Work out the finished part from the listing and answer in its coordinate system (mm). A direction names the side the tool comes from. Give positions to 0.01 mm unless a question says otherwise; leave off trailing zeros. Loops run counter-clockwise (first coordinate to the right, second up) from the corner with the lowest first, then second, coordinate; pieces in that order, holes last. Notation, with made-up numbers: M 58,13.25 L 87,13.25 A26 ccw 87,28.25 Z; hole C 58,12 d5. An arc over 180 degrees is marked long. Answer in a Markdown table with one row per item. Add a question column.
from build123d import *

# Parameters (mm, degrees)
F0_W      = 131
F0_H      = 59
F0_W_2    = 85
F0_H_2    = 55
F0_W_3    = 40
F1_DEPTH  = 22
F2_W      = 40
F2_H      = 2
F3_DEPTH  = 55
F4_W      = 85
F4_H      = 3.4782900475
F5_DEPTH  = 55
F7_DEPTH  = 2
F8_R      = 2
F9_DEPTH  = 2
F10_R     = 4
F11_DEPTH = 20
F12_DEPTH = 20
F13_R     = 4
F14_R     = 6.25
F15_DEPTH = 25


with BuildPart() as f1:
    # F0 (on Top) → F1 (new body)
    with BuildSketch(Plane.XY):
        Rectangle(F0_W, F0_H)
        with Locations((-21, 0)):
            Rectangle(F0_W_2, F0_H_2, mode=Mode.SUBTRACT)
        with Locations((43.5, 0)):
            Rectangle(F0_W_3, F0_H_2, mode=Mode.SUBTRACT)
    extrude(amount=F1_DEPTH)

    # F2 (on face) → F3 (join)
    with BuildSketch(Plane.XZ.offset(-27.5)):
        with Locations((43.5, 21)):
            Rectangle(F2_W, F2_H)
    extrude(amount=F3_DEPTH)

    # F4 (on face) → F5 (join)
    with BuildSketch(Plane.XZ.offset(-27.5)):
        with Locations((-21, 1.7391450237)):
            Rectangle(F4_W, F4_H)
    extrude(amount=F5_DEPTH)

    # F6 (on face) → F7 (join)
    with BuildSketch(Plane.XY.offset(22)):
        Polygon((21.5, -29.5), (65.5, -29.5), (65.5, 29.5), (21.5, 29.5), (21.5, 27.5), (21.5, -27.5), align=None)
    extrude(amount=F7_DEPTH)

    # F8 (on face) → F9 (cut)
    with BuildSketch(Plane(origin=(21.5, 0, 0), x_dir=(0, -1, 0), z_dir=(-1, 0, 0))):
        with Locations((0, 10.4782900475)):
            Circle(F8_R)
    extrude(amount=-F9_DEPTH, mode=Mode.SUBTRACT)

    # F10
    f10_edges = [f1.edges().sort_by_distance(p)[0] for p in [
        (65.5, -29.5, 12),
        (65.5, 29.5, 12),
        (63.5, -27.5, 10),
        (63.5, 27.5, 10),
    ]]
    fillet(f10_edges, radius=F10_R)

    # F11 (add): a face of the model
    f11_faces = [f1.faces().sort_by_distance(p)[0] for p in [
        (-65.5, 0, 11),
    ]]
    extrude(f11_faces, amount=F11_DEPTH)

    # F12 (cut): a face of the model
    f12_faces = [f1.faces().sort_by_distance(p)[0] for p in [
        (-63.5, 0, 12.7391450237),
    ]]
    extrude(f12_faces, amount=-F12_DEPTH, mode=Mode.SUBTRACT)

    # F13
    f13_edges = [f1.edges().sort_by_distance(p)[0] for p in [
        (-83.5, 27.5, 12.739145),
        (-85.5, -29.5, 11),
        (-83.5, -27.5, 12.739145),
        (-85.5, 29.5, 11),
    ]]
    fillet(f13_edges, radius=F13_R)

    # F14 (on face) → F15 (cut)
    with BuildSketch(Plane(origin=(-85.5, 0, 0), x_dir=(0, -1, 0), z_dir=(-1, 0, 0))):
        with Locations((0, 11)):
            Circle(F14_R)
    extrude(amount=-F15_DEPTH, mode=Mode.SUBTRACT)


solid = f1.part
(1) The mould has two halves that part along X. Classify faces 5 (the face through (64.297, -28.359, 12.168)), 6 (the face through (-32, 0, 3.478)), 7 (the face through (-85.5, -6, 8)): pulls with the +X half, pulls with the -X half, needs draft (parallel to the pull), parting line crosses it, or undercut.
(2) Each of these flat-tipped pins is pushed along its axis until it touches: P1, Ø1.5, axis at x = 32, y = -4.5, coming from the -Z side; P2, Ø3.5, axis at y = 0, z = 10.48, coming from the -X side. Where does it stop, or does it pass through?
(3) Which of the six approach directions +Z, -Z, +X, -X, +Y, -Y give full straight-line access (tool end or side, diameter ignored) to faces 1 (the face through (-84.297, -28.359, 11.154)), 2 (the face through (-32, 28, 22)), 3 (the face through (-28, 27.5, 13)), 4 (the face through (63.5, 0, 10))?
(4) Section C-C, the plane x = -18 is taken. Determine the outline of the cut face in (y, z), and give its area (3 significant figures).
(5) Section A-A, the plane y = 0 is taken. Determine the outline of the cut face in (x, z), and give its area (3 significant figures).
(6) Consider line 1 along X through (y, z) = (-15.5, 4.5); line 2 along Y through (x, z) = (45, 5.25); line 3 along Z through (x, y) = (22.1, 0). Determine where each line is inside the solid, lowest interval first. Write a range as from..to.
(7) Section B-B, the plane y = -14 is taken. Determine the outline of the cut face in (x, z).
Numbers:
| question | item | result |
|---|---|---|
| 1 | face 5 | pulls with the +X half |
| 1 | face 6 | undercut |
| 1 | face 7 | pulls with the -X half |
| 2 | P1 | stops at z = 20 |
| 2 | P2 | stops at x = 63.5 |
| 3 | face 1 | +Z, -Z, -X, -Y |
| 3 | face 2 | +Z, -X, +Y, -Y |
| 3 | face 3 | +Z |
| 3 | face 4 | -Z |
| 4 | outline | M -29.5,0 L 29.5,0 L 29.5,22 L 27.5,22 L 27.5,3.48 L -27.5,3.48 L -27.5,22 L -29.5,22 Z |
| 4 | area | 279 mm² |
| 5 | outline | M -85.5,0 L 23.5,0 L 23.5,8.48 L 21.5,8.48 L 21.5,3.48 L -83.5,3.48 L -83.5,4.75 L -85.5,4.75 Z; M -85.5,17.25 L -83.5,17.25 L -83.5,22 L -85.5,22 Z; M 21.5,12.48 L 23.5,12.48 L 23.5,20 L 63.5,20 L 63.5,0 L 65.5,0 L 65.5,24 L 21.5,24 Z |
| 5 | area | 632 mm² |
| 6 | line 1 | x = -85.5..-83.5, 21.5..23.5, 63.5..65.5 |
| 6 | line 2 | y = -29.5..-27.5, 27.5..29.5 |
| 6 | line 3 | z = 0..8.48, 12.48..24 |
| 7 | outline | M -85.5,0 L 23.5,0 L 23.5,20 L 63.5,20 L 63.5,0 L 65.5,0 L 65.5,24 L 21.5,24 L 21.5,3.48 L -83.5,3.48 L -83.5,22 L -85.5,22 Z |
